```python
from build123d import *

# Parameters (mm, degrees)
SKETCH1_W           = 24.999989911
SKETCH1_H           = 10.457138346
SKETCH1_W_2         = 49.999979698
SKETCH1_H_2         = 10.999995004
BOSS_EXTRUDE1_DEPTH = 6


with BuildPart() as part:
    # Sketch1 → Boss-Extrude1 (new body)
    with BuildSketch(Plane.XY):
        Polygon((-13.869587182, 182.416079474), (-65.562023318, 182.416079474), (-70.562021318, 187.416077474), (-70.562021318, 253.330336135), (-65.562023318, 258.330334135), (-13.869587203, 258.330334135), (-8.86958931, 253.330336243), (-8.869589201, 187.416077455), align=None)
        with Locations((-39.715805198, 197.994644352)):
            Rectangle(SKETCH1_W, SKETCH1_H, mode=Mode.SUBTRACT)
        with Locations((-39.71580491, 243.023197048)):
            Rectangle(SKETCH1_W_2, SKETCH1_H_2, mode=Mode.SUBTRACT)
        Polygon((-64.027895433, 218.634541052), (-63.562021338, 218.573207564), (-63.096147243, 218.634541052), (-62.662021698, 218.81436174), (-62.289229641, 219.100415147), (-62.003176235, 219.473207204), (-61.823355546, 219.907332749), (-61.762022058, 220.373206844), (-61.823355546, 220.839080938), (-62.003176235, 221.273206484), (-62.289229641, 221.645998541), (-62.662021698, 221.932051947), (-63.096147243, 222.111872635), (-63.562021338, 222.173206124), (-64.027895433, 222.111872635), (-64.462020978, 221.932051947), (-64.834813035, 221.645998541), (-65.120866442, 221.273206484), (-65.30068713, 220.839080938), (-65.362020618, 220.373206844), (-65.30068713, 219.907332749), (-65.120866442, 219.473207204), (-64.834813035, 219.100415147), (-64.462020978, 218.81436174), align=None, mode=Mode.SUBTRACT)
        Polygon((-15.869589261, 222.173206124), (-16.335463356, 222.111872635), (-16.769588901, 221.932051947), (-17.142380958, 221.645998541), (-17.428434364, 221.273206484), (-17.608255053, 220.839080938), (-17.669588541, 220.373206844), (-17.608255053, 219.907332749), (-17.428434364, 219.473207204), (-17.142380958, 219.100415147), (-16.769588901, 218.81436174), (-16.335463356, 218.634541052), (-15.869589261, 218.573207564), (-15.403715166, 218.634541052), (-14.969589621, 218.81436174), (-14.596797564, 219.100415147), (-14.310744158, 219.473207204), (-14.130923469, 219.907332749), (-14.069589981, 220.373206844), (-14.130923469, 220.839080938), (-14.310744158, 221.273206484), (-14.596797564, 221.645998541), (-14.969589621, 221.932051947), (-15.403715166, 222.111872635), align=None, mode=Mode.SUBTRACT)
        Polygon((-37.977139428, 187.881953608), (-38.156960116, 188.316079153), (-38.443013523, 188.68887121), (-38.81580558, 188.974924616), (-39.249931125, 189.154745305), (-39.71580522, 189.216078793), (-40.181679314, 189.154745305), (-40.61580486, 188.974924616), (-40.988596917, 188.68887121), (-41.274650323, 188.316079153), (-41.454471012, 187.881953608), (-41.5158045, 187.416079513), (-41.454471012, 186.950205418), (-41.274650323, 186.516079873), (-40.988596917, 186.143287816), (-40.61580486, 185.857234409), (-40.181679314, 185.677413721), (-39.71580522, 185.616080233), (-39.249931125, 185.677413721), (-38.81580558, 185.857234409), (-38.443013523, 186.143287816), (-38.156960116, 186.516079873), (-37.977139428, 186.950205418), (-37.91580594, 187.416079513), align=None, mode=Mode.SUBTRACT)
        Polygon((-37.977139428, 252.86446006), (-37.91580594, 253.330334155), (-37.977139428, 253.79620825), (-38.156960116, 254.230333795), (-38.443013523, 254.603125852), (-38.81580558, 254.889179258), (-39.249931125, 255.068999947), (-39.71580522, 255.130333435), (-40.181679314, 255.068999947), (-40.61580486, 254.889179258), (-40.988596917, 254.603125852), (-41.274650323, 254.230333795), (-41.454471012, 253.79620825), (-41.5158045, 253.330334155), (-41.454471012, 252.86446006), (-41.274650323, 252.430334515), (-40.988596917, 252.057542458), (-40.61580486, 251.771489052), (-40.181679314, 251.591668363), (-39.71580522, 251.530334875), (-39.249931125, 251.591668363), (-38.81580558, 251.771489052), (-38.443013523, 252.057542458), (-38.156960116, 252.430334515), align=None, mode=Mode.SUBTRACT)
    extrude(amount=BOSS_EXTRUDE1_DEPTH)


solid = part.part
```
Check sheet for the modelled part. Datum: model origin and axes. Units: mm. A direction names the side the tool comes from. Give positions to 0.01 mm unless a question says otherwise; leave off trailing zeros. Write each loop counter-clockwise with the first axis right and the second up, starting at its lowest first coordinate (ties: lowest second). Pieces come first, ordered by that corner, then holes. Notation, with made-up numbers: (85, 73.5) - (143, 73.5) arc R19 ccw to (143, 104.5) - close; hole circle Ø6 at (-5.75, 60). An arc over 180 degrees is marked (long way). Answer as a JSON object with one key per item and string values. Group by question number.
1) Access from +Z, -Z, +X, -X, +Y, -Y to the whole of each face (thin tool, end or side, straight path). Record for faces 5 (the face through (-27.216, 198, 3)), 6 (the face through (-70.562, 220, 3)).
2) Sectioned sample at A-A (x = -23.5). Record the cut outline in (y, z), then the cut area to 3 significant figures.
3) Sectioned sample at B-B (y = 196.5). Record the cut outline in (x, z).
4) Release check for a two-part mould opening along Y. For faces 1 (the face through (-11.335, 184.951, 2.958)), 2 (the face through (-40, 203.223, 3)), 3 (the face through (-8.87, 221, 3)), 4 (the face through (-40, 258.33, 3)) record: pulls with the +Y half, pulls with the -Y half, needs draft (parallel to the pull), parting line crosses it, or undercut.
5) Sectioned sample at C-C (z = 5.2). Give the number of separate pieces and of enclosed holes in the cut face, then the cut area to 3 significant figures.
6) Thickness scan on probe 1 along Y at (x, z) = (-35, 2.8); probe 2 along X at (y, z) = (242, 5.7); probe 3 along Y at (x, z) = (-26.5, 5.75). Record the ranges inside material, lowest first. Write a range as from..to.
Geometry results:
{
 "1": {"face 5": "+Z, -Z", "face 6": "+Z, -Z, -X, +Y, -Y"},
 "2": {"outline": "(182.42, 0) - (237.52, 0) - (237.52, 6) - (182.42, 6) - close; (248.52, 0) - (258.33, 0) - (258.33, 6) - (248.52, 6) - close", "area": "389 mm^2"},
 "3": {"outline": "(-70.56, 0) - (-52.22, 0) - (-52.22, 6) - (-70.56, 6) - close; (-27.22, 0) - (-8.87, 0) - (-8.87, 6) - (-27.22, 6) - close"},
 "4": {"face 1": "pulls with the -Y half", "face 2": "undercut", "face 3": "needs draft", "face 4": "pulls with the +Y half"},
 "5": {"separate pieces": "1", "enclosed holes": "6", "area": "3,780 mm^2"},
 "6": {"probe 1": "y = 182.42..192.77, 203.22..237.52, 248.52..258.33", "probe 2": "x = -70.56..-64.72, -14.72..-8.87", "probe 3": "y = 182.42..237.52, 248.52..258.33"}
}
